Read the model definition and answer for the solid it produces. Units are mm, in the model's axes. Face numbers are marked on the shaded views. A direction names the side the tool comes from. Give positions to 0.01 mm unless a question says otherwise; leave off trailing zeros. Write each loop counter-clockwise with the first axis right and the second up, starting at its lowest first coordinate (ties: lowest second). Pieces come first, ordered by that corner, then holes. Notation, with made-up numbers: (5, 36) -> (55, 36) arc R27 ccw to (55, 67) -> close; hole circle Ø3 at (38, -37). An arc over 180 degrees is marked (long way). Write item = value, one per line.
from build123d import *

# Parameters (mm, degrees)
F0_R      = 32.5
F1_DEPTH  = 25
F2_R      = 22.5
F3_DEPTH  = 25
F4_R      = 20
F5_DEPTH  = 15
F6_R      = 15
F7_DEPTH  = 20
F9_W      = 24
F9_H      = 30
F10_DEPTH = 100
F8_R      = 7.5
F12_DEPTH = 25


with BuildPart() as f1:
    # F0 (on Front) → F1 (new body)
    with BuildSketch(Plane.XZ):
        with Locations((-32.571085, 33.19031)):
            Circle(F0_R)
    extrude(amount=F1_DEPTH)

    # F2 (on face) → F3 (join)
    with BuildSketch(Plane.XZ.offset(25)):
        with Locations((-32.571085, 33.19031)):
            Circle(F2_R)
    extrude(amount=F3_DEPTH)

    # F4 (on face) → F5 (cut)
    with BuildSketch(Plane(origin=(0, 0, 0), x_dir=(-1, 0, 0), z_dir=(0, 1, 0))):
        with Locations((32.571085, 33.19031)):
            Circle(F4_R)
    extrude(amount=-F5_DEPTH, mode=Mode.SUBTRACT)

    # F6 (on face) → F7 (cut)
    with BuildSketch(Plane(origin=(0, -15, 0), x_dir=(-1, 0, 0), z_dir=(0, 1, 0))):
        with Locations((32.571085, 33.19031)):
            Circle(F6_R)
    extrude(amount=-F7_DEPTH, mode=Mode.SUBTRACT)

    # F9 (on Top) → F10 (cut)
    with BuildSketch(Plane.XY):
        with Locations((-32, -15)):
            Rectangle(F9_W, F9_H)
    extrude(amount=F10_DEPTH, mode=Mode.SUBTRACT)

    # F8 (on face) → F12 (cut)
    with BuildSketch(Plane(origin=(0, -35, 0), x_dir=(-1, 0, 0), z_dir=(0, 1, 0))):
        with Locations((32.571085, 33.19031)):
            Circle(F8_R)
    extrude(amount=-F12_DEPTH, mode=Mode.SUBTRACT)


solid = f1.part
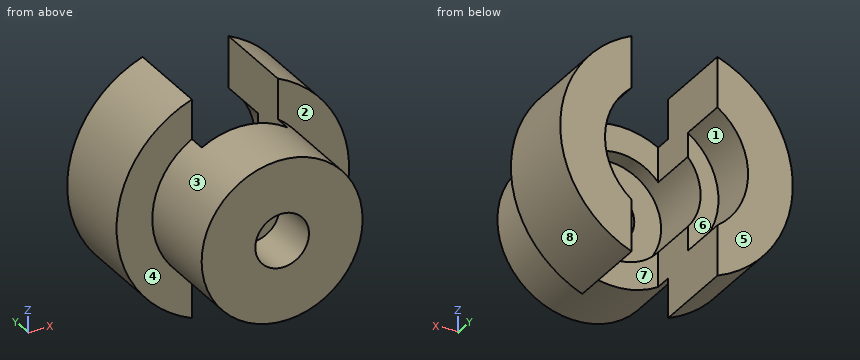
(1) The part is cut by section D-D on z = 46. Determine the outline of the cut face in (x, y).
Checks:
outline = (-62.44, -25) -> (-51.07, -25) -> (-51.07, -50) -> (-14.07, -50) -> (-14.07, -25) -> (-2.7, -25) -> (-2.7, 0) -> (-17.21, 0) -> (-17.21, -15) -> (-20, -15) -> (-20, -30) -> (-24.77, -30) -> (-24.77, -35) -> (-40.38, -35) -> (-40.38, -30) -> (-44, -30) -> (-44, -15) -> (-47.93, -15) -> (-47.93, 0) -> (-62.44, 0) -> close
(2) The part is cut by section C-C on z = 9. Determine the outline of the cut face in (x, y).
Checks:
outline = (-54.28, -25) -> (-44, -25) -> (-44, 0) -> (-54.28, 0) -> close; (-20, -25) -> (-10.87, -25) -> (-10.87, 0) -> (-20, 0) -> close
(3) The part is cut by section A-A on y = -10. Determine the outline of the cut face in (x, z) (3 decimals), plus the area to 3 significant figures.
Checks:
outline = (-44, 2.766) -> (-44, 16.778) arc R20 cw to (-44, 49.603) -> (-44, 63.614) arc R32.5 ccw to start; (-20, 3.22) arc R32.5 ccw to (-20, 63.161) -> (-20, 48.746) arc R20 cw to (-20, 17.635) -> close
area = 1,440 mm²
(4) For a pull along Z with two mould halves and no side action, classify the marked faces 1, 2 and 3 as released by +Z, released by -Z, zero draft, split by the parting line, or undercut.
Checks:
face_1 = undercut
face_2 = zero draft
face_3 = split by the parting line
(5) Given P1, Ø11, axis at y = -16.5, z = 54, coming from the -X side; P2, Ø7, axis at x = -34, z = 50, coming from the +Y side; P3, Ø6, axis at y = -18.5, z = 10, coming from the +X side, each flat-ended and moving along its own axis, determine where each tip first touches the part or whether it passes through.
Checks:
P1 = -61.24
P2 = -30
P3 = -7.1
(6) The part is cut by section B-B on x = -33. Determine the outline of the cut face in (y, z), plus the area to 3 significant figures.
Checks:
outline = (-50, 10.69) -> (-30, 10.69) -> (-30, 18.2) -> (-35, 18.2) -> (-35, 25.7) -> (-50, 25.7) -> close; (-50, 40.68) -> (-35, 40.68) -> (-35, 48.18) -> (-30, 48.18) -> (-30, 55.69) -> (-50, 55.69) -> close
area = 525 mm²
(7) Consider L1, parallel to X at y = -31, z = 33.5; L2, parallel to Y at x = -36, z = 23; L3, parallel to X at y = -7.5, z = 7.5. Determine where each line is inside the solid, lowest interval first.
Checks:
L1 = -55.07 to -47.57, -17.57 to -10.07
L2 = -50 to -35
L3 = -52.48 to -44, -20 to -12.66
(8) A tool of negligible diameter and unlimited length cuts with its end or side. For the marked faces 4, 5, 6, 7 and 8, from which of +Z, -Z, +X, -X, +Y, -Y can it reach the whole face along a straight path? Write none if from no direction.
Checks:
face_4 = -X, -Y
face_5 = +Z, -Z, +X, -X, +Y
face_6 = +Y
face_7 = +Z, -Z, +Y
face_8 = +X, +Y, -Y
